```python
from build123d import *

# Parameters (mm, degrees)
SKETCH_1_W          = 200
SKETCH_1_H          = 120
EXTRUDE_1_DEPTH     = 100
SKETCH_2_W          = 184
SKETCH_2_H          = 104
CUT_EXTRUDE_1_DEPTH = 90
SKETCH_3_R          = 35
EXTRUDE_2_DEPTH     = 20
EXTRUDE_START       = -20
SKETCH_4_R          = 35
EXTRUDE_3_DEPTH     = 20
SKETCH_5_W          = 8
SKETCH_5_H          = 25
EXTRUDE_4_DEPTH     = 20
SKETCH_6_W          = 8
SKETCH_6_H          = 25
EXTRUDE_5_DEPTH     = 20
SKETCH_7_W          = 30
SKETCH_7_H          = 120
EXTRUDE_6_DEPTH     = 12
SKETCH_8_W          = 240
SKETCH_8_H          = 160
SKETCH_8_W_2        = 184
SKETCH_8_H_2        = 104
EXTRUDE_7_DEPTH     = 10
SKETCH_9_R          = 5.5
CUT_EXTRUDE_2_DEPTH = 10
SKETCH_10_R         = 23.5
CUT_EXTRUDE_3_DEPTH = 226.665681928
SKETCH_11_R         = 26
CUT_EXTRUDE_4_DEPTH = 226.665681928
SKETCH_12_R         = 5.1
CUT_EXTRUDE_5_DEPTH = 10
SKETCH_14_R         = 6.5
CUT_EXTRUDE_7_DEPTH = 12
SKETCH_15_R         = 7
CUT_EXTRUDE_8_DEPTH = 8


with BuildPart() as part:
    # 草图1 → 凸台-拉伸1 (new body)
    with BuildSketch(Plane.XY):
        Rectangle(SKETCH_1_W, SKETCH_1_H)
    extrude(amount=EXTRUDE_1_DEPTH)

    # 草图2 → 切除-拉伸1 (cut)
    with BuildSketch(Plane.XY.offset(10)):
        Rectangle(SKETCH_2_W, SKETCH_2_H)
    extrude(amount=CUT_EXTRUDE_1_DEPTH, mode=Mode.SUBTRACT)

    # 草图3 → 凸台-拉伸2 (add)
    with BuildSketch(Plane(origin=(0, 55, 0), x_dir=(1, 0, 0), z_dir=(0, 1, 0))):
        with Locations(Location((-45, -50, 0), (0, 0, 90))):
            Circle(SKETCH_3_R)
        with Locations(Location((50, -50, 0), (0, 0, 90))):
            Circle(SKETCH_3_R)
    extrude(amount=EXTRUDE_2_DEPTH)

    # 草图4 → 凸台-拉伸3 (add)
    with BuildSketch(Plane(origin=(0, -55, 0), x_dir=(1, 0, 0), z_dir=(0, 1, 0)).offset(EXTRUDE_START)):
        with Locations(Location((-45, -50, 0), (0, 0, 90))):
            Circle(SKETCH_4_R)
        with Locations(Location((50, -50, 0), (0, 0, 90))):
            Circle(SKETCH_4_R)
    extrude(amount=EXTRUDE_3_DEPTH)

    # 草图5 → 凸台-拉伸4 (add)
    with BuildSketch(Plane(origin=(0, 55, 0), x_dir=(1, 0, 0), z_dir=(0, 1, 0))):
        with Locations((-45, -12.5)):
            Rectangle(SKETCH_5_W, SKETCH_5_H)
        with Locations((50, -12.5)):
            Rectangle(SKETCH_5_W, SKETCH_5_H)
    extrude(amount=EXTRUDE_4_DEPTH)

    # 草图6 → 凸台-拉伸5 (add)
    with BuildSketch(Plane(origin=(0, -55, 0), x_dir=(1, 0, 0), z_dir=(0, 1, 0))):
        with Locations((-45, -12.5)):
            Rectangle(SKETCH_6_W, SKETCH_6_H)
        with Locations((50, -12.5)):
            Rectangle(SKETCH_6_W, SKETCH_6_H)
    extrude(amount=-EXTRUDE_5_DEPTH)

    # 草图7 → 凸台-拉伸6 (add)
    with BuildSketch(Plane.XY):
        with Locations((115, 0)):
            Rectangle(SKETCH_7_W, SKETCH_7_H)
        with Locations((-115, 0)):
            Rectangle(SKETCH_7_W, SKETCH_7_H)
    extrude(amount=EXTRUDE_6_DEPTH)

    # 草图8 → 凸台-拉伸7 (add)
    with BuildSketch(Plane.XY.offset(90)):
        Rectangle(SKETCH_8_W, SKETCH_8_H)
        Rectangle(SKETCH_8_W_2, SKETCH_8_H_2, mode=Mode.SUBTRACT)
    extrude(amount=EXTRUDE_7_DEPTH)

    # 草图9 → 切除-拉伸2 (cut)
    with BuildSketch(Plane.XY.offset(90)):
        with Locations((-110, 70)):
            Circle(SKETCH_9_R)
        with Locations((110, 70)):
            Circle(SKETCH_9_R)
        with Locations((-110, -70)):
            Circle(SKETCH_9_R)
        with Locations((110, -70)):
            Circle(SKETCH_9_R)
        with Locations((0, 70)):
            Circle(SKETCH_9_R)
        with Locations((0, -70)):
            Circle(SKETCH_9_R)
    extrude(amount=CUT_EXTRUDE_2_DEPTH, mode=Mode.SUBTRACT)

    # 草图10 → 切除-拉伸3 (cut, through all)
    with BuildSketch(Plane(origin=(0, 75, 0), x_dir=(1, 0, 0), z_dir=(0, 1, 0))):
        with Locations(Location((-45, -50, 0), (0, 0, 270))):
            Circle(SKETCH_10_R)
    extrude(amount=-CUT_EXTRUDE_3_DEPTH, mode=Mode.SUBTRACT)

    # 草图11 → 切除-拉伸4 (cut, through all)
    with BuildSketch(Plane(origin=(0, 75, 0), x_dir=(1, 0, 0), z_dir=(0, 1, 0))):
        with Locations(Location((50, -50, 0), (0, 0, 270))):
            Circle(SKETCH_11_R)
    extrude(amount=-CUT_EXTRUDE_4_DEPTH, mode=Mode.SUBTRACT)

    # 草图12 → 切除-拉伸5 (cut)
    with BuildSketch(Plane.XY):
        Circle(SKETCH_12_R)
    extrude(amount=CUT_EXTRUDE_5_DEPTH, mode=Mode.SUBTRACT)

    # 草图14 → 切除-拉伸7 (cut)
    with BuildSketch(Plane.XY):
        with Locations((115, 40)):
            Circle(SKETCH_14_R)
        with Locations((115, -40)):
            Circle(SKETCH_14_R)
        with Locations((-115, 40)):
            Circle(SKETCH_14_R)
        with Locations((-115, -40)):
            Circle(SKETCH_14_R)
    extrude(amount=CUT_EXTRUDE_7_DEPTH, mode=Mode.SUBTRACT)

    # 草图15 → 切除-拉伸8 (cut)
    with BuildSketch(Plane(origin=(100, 0, 0), x_dir=(0, 0, -1), z_dir=(1, 0, 0))):
        with Locations((-40, 0)):
            Circle(SKETCH_15_R)
    extrude(amount=-CUT_EXTRUDE_8_DEPTH, mode=Mode.SUBTRACT)


solid = part.part
```
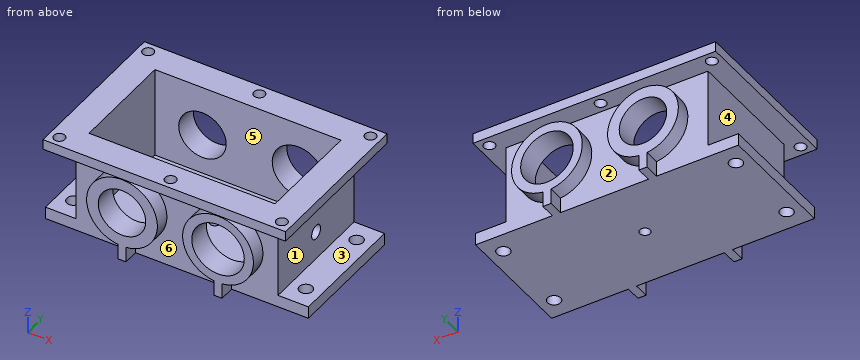
The model under review builds one solid part; all positions refer to its coordinate system, in mm. Face numbers are marked on the shaded views. A direction names the side the tool comes from. Give positions to 0.01 mm unless a question says otherwise; leave off trailing zeros. Write each loop counter-clockwise with the first axis right and the second up, starting at its lowest first coordinate (ties: lowest second). Pieces come first, ordered by that corner, then holes. Notation, with made-up numbers: (59.5, 51.25) -> (64.5, 51.25) arc R34 cw to (64.5, 85.25) -> close; hole circle Ø11 at (9, 47). An arc over 180 degrees is marked (long way). Answer in a Markdown table with one row per item.
1) Add section D-D on x = 0. State the section outline as (y, z) points.
Worked answers:
| item | result |
|---|---|
| outline | (-80, 90) -> (-75.5, 90) -> (-75.5, 100) -> (-80, 100) -> close; (-64.5, 90) -> (-60, 90) -> (-60, 0) -> (-5.1, 0) -> (-5.1, 10) -> (-52, 10) -> (-52, 100) -> (-64.5, 100) -> close; (5.1, 0) -> (60, 0) -> (60, 90) -> (64.5, 90) -> (64.5, 100) -> (52, 100) -> (52, 10) -> (5.1, 10) -> close; (75.5, 90) -> (80, 90) -> (80, 100) -> (75.5, 100) -> close |
2) Mouldability with a two-part tool opening along X and no side actions: class the marked faces 1, 2 and 3 as +X half, -X half, draft (parallel to the pull), parting line (faces both ways), or undercut.
Worked answers:
| item | result |
|---|---|
| face 1 | +X half |
| face 2 | undercut |
| face 3 | draft |
3) Add section B-B on x = -45. State the section outline as (y, z) points.
Worked answers:
| item | result |
|---|---|
| outline | (-80, 90) -> (-60, 90) -> (-60, 85) -> (-75, 85) -> (-75, 73.5) -> (-52, 73.5) -> (-52, 100) -> (-80, 100) -> close; (-75, 0) -> (75, 0) -> (75, 26.5) -> (52, 26.5) -> (52, 10) -> (-52, 10) -> (-52, 26.5) -> (-75, 26.5) -> close; (52, 73.5) -> (75, 73.5) -> (75, 85) -> (60, 85) -> (60, 90) -> (80, 90) -> (80, 100) -> (52, 100) -> close |
4) Tool access review of the marked faces 4, 5 and 6: name each direction out of +Z, -Z, +X, -X, +Y, -Y from which nothing blocks a thin tool from reaching the whole face with its end or side.
Worked answers:
| item | result |
|---|---|
| face 4 | -X, +Y, -Y |
| face 5 | +Z |
| face 6 | -Y |
5) For L1, parallel to Y at x = -110, z = 94; L2, parallel to X at y = -67, z = 50; L3, parallel to Y at x = 16, z = 59.5, list the stretches that pass through material, from the lowest coordinate up. Write a range as [from, to].
Worked answers:
| item | result |
|---|---|
| L1 | [-80, -75.5], [-64.5, 64.5], [75.5, 80] |
| L2 | [-80, -68.5], [-21.5, -10], [15, 24], [76, 85] |
| L3 | [-60, -52], [52, 60] |
6) Add section A-A on y = -70. State the section outline as (x, z) points, plus the area to 3 significant figures.
Worked answers:
| item | result |
|---|---|
| outline | (-120, 90) -> (-115.5, 90) -> (-115.5, 100) -> (-120, 100) -> close; (-104.5, 90) -> (-5.5, 90) -> (-5.5, 100) -> (-104.5, 100) -> close; (-49, 0) -> (-41, 0) -> (-41, 15.23) arc R35 ccw (long way) to (-49, 15.23) -> close; (5.5, 90) -> (104.5, 90) -> (104.5, 100) -> (5.5, 100) -> close; (46, 0) -> (54, 0) -> (54, 15.23) arc R35 ccw (long way) to (46, 15.23) -> close; (115.5, 90) -> (120, 90) -> (120, 100) -> (115.5, 100) -> close; hole circle Ø47 at (-45, 50); hole circle Ø52 at (50, 50) |
| area | 6,150 mm² |
7) Clearance check with flat-ended pins moving along their axes: P1, Ø4, axis at x = -86.5, z = 27, coming from the -Y side; P2, Ø8, axis at y = -18.5, z = 41, coming from the -X side; P3, Ø12, axis at y = 69, z = 7, coming from the -X side. State where each tip first meets the part, or that it passes through.
Worked answers:
| item | result |
|---|---|
| P1 | y = -60 |
| P2 | x = -100 |
| P3 | x = -49 |
8) Add section C-C on y = 0. State the section outline as (x, z) points.
Worked answers:
| item | result |
|---|---|
| outline | (-130, 0) -> (-5.1, 0) -> (-5.1, 10) -> (-92, 10) -> (-92, 100) -> (-120, 100) -> (-120, 90) -> (-100, 90) -> (-100, 12) -> (-130, 12) -> close; (5.1, 0) -> (130, 0) -> (130, 12) -> (100, 12) -> (100, 33) -> (92, 33) -> (92, 10) -> (5.1, 10) -> close; (92, 47) -> (100, 47) -> (100, 90) -> (120, 90) -> (120, 100) -> (92, 100) -> close |
